Verification items for this drawing (mm, ordinates from the low corner). Give positions to 0.01 mm unless a question says otherwise; leave off trailing zeros. Order: outer loops, then holes, each group sorted by start corner. A loop starts at its lowest first (then second) coordinate and runs counter-clockwise, first axis right, second up. Notation, with made-up numbers: (-31, 34) -> (2, 34) arc R19 ccw to (2, 52) -> close; hole circle Ø1 at (1.5, 81). An arc over 180 degrees is marked (long way). One line per question, with ' | ' between items.
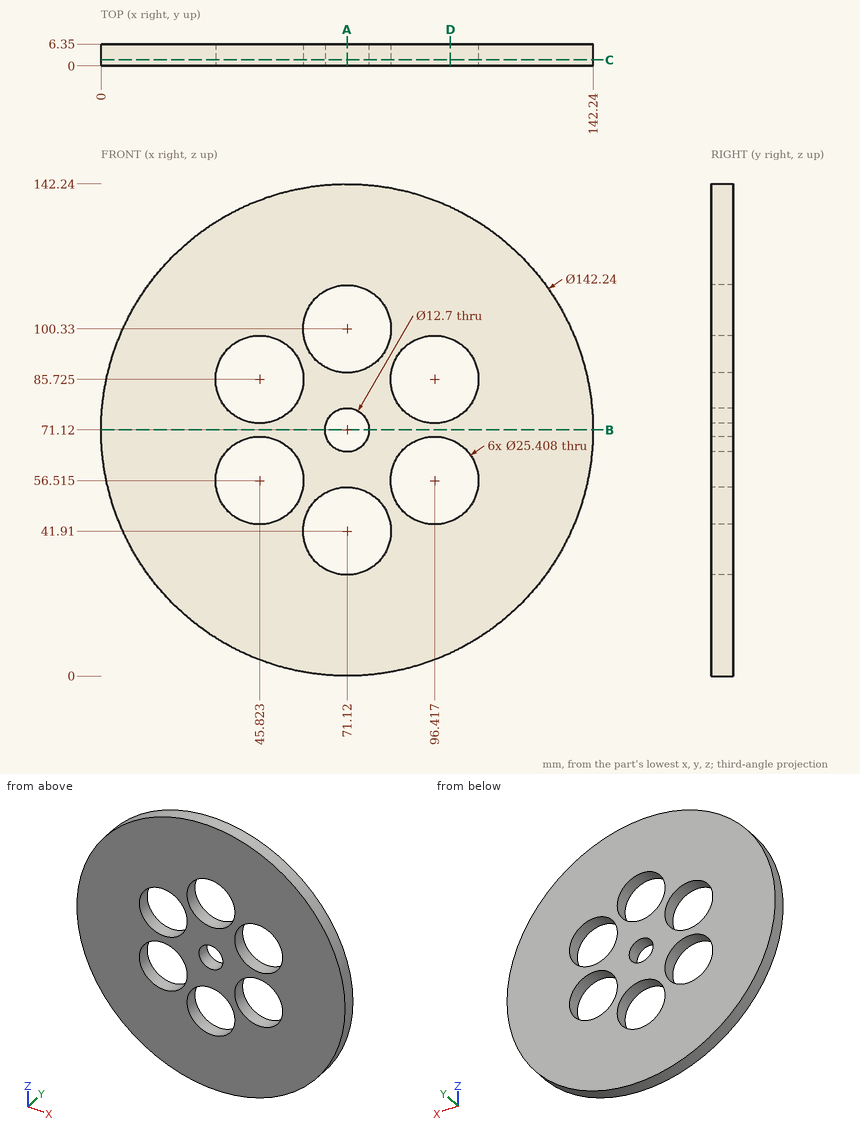
Q1. Section check B-B (z = 71.12). Enter the section's corners in (x, y).
Result sheet:
outline: (0, 0) -> (64.77, 0) -> (64.77, 6.35) -> (0, 6.35) -> close; (77.47, 0) -> (142.24, 0) -> (142.24, 6.35) -> (77.47, 6.35) -> close
Q2. Depth check by flat-ended pin: pin 1 Ø12 at (x, z) = (81.5, 38.5) entering from -Y; pin 2 Ø8 at (x, z) = (94.5, 61) entering from -Y; pin 3 Ø3 at (x, y) = (74.5, 4) entering from -Z (1 decimal); pin 4 Ø1.5 at (y, z) = (1, 97) entering from -X. Enter the tip coordinate at first touch or a pass-through.
Result sheet:
pin 1: stops at y = 0 | pin 2: passes through | pin 3: stops at z = 0 | pin 4: stops at x = 4.59
Q3. Thickness scan on line 1 (Z direction, x = 71.12, y = 1.75); line 2 (X direction, y = 1.25, z = 92) (1 decimal); line 3 (X direction, y = 6, z = 94) (1 decimal). Record the ranges inside material, lowest first.
Result sheet:
line 1: z = 0 to 29.21, 54.61 to 64.77, 77.47 to 87.63, 113.03 to 142.24 | line 2: x = 3.1 to 34.8, 56.9 to 61.5, 80.7 to 85.4, 107.5 to 139.1 | line 3: x = 3.8 to 36.2, 55.5 to 60.1, 82.1 to 86.8, 106.1 to 138.5
Q4. Section check D-D (x = 101). Enter the section's corners in (y, z), and give its area (3 significant figures).
Result sheet:
outline: (0, 6.58) -> (6.35, 6.58) -> (6.35, 44.67) -> (0, 44.67) -> close; (0, 68.36) -> (6.35, 68.36) -> (6.35, 73.88) -> (0, 73.88) -> close; (0, 97.57) -> (6.35, 97.57) -> (6.35, 135.66) -> (0, 135.66) -> close | area: 519 mm2
Q5. Section check C-C (y = 1.75). Count the separate pieces of the cut face and the enclosed holes in it, and give its area (3 significant figures).
Result sheet:
separate pieces: 1 | enclosed holes: 7 | area: 12,700 mm2
Q6. Section check A-A (x = 71.12). Enter the section's corners in (y, z), and give its area (3 significant figures).
Result sheet:
outline: (0, 0) -> (6.35, 0) -> (6.35, 29.21) -> (0, 29.21) -> close; (0, 54.61) -> (6.35, 54.61) -> (6.35, 64.77) -> (0, 64.77) -> close; (0, 77.47) -> (6.35, 77.47) -> (6.35, 87.63) -> (0, 87.63) -> close; (0, 113.03) -> (6.35, 113.03) -> (6.35, 142.24) -> (0, 142.24) -> close | area: 500 mm2
